```python
from build123d import *

# Parameters (mm, degrees)
BOSS_EXTRUDE1_DEPTH = 10.414
CUT_EXTRUDE1_DEPTH  = 6.08
CUT_EXTRUDE3_DEPTH  = 2.38125
CUT_EXTRUDE2_DEPTH  = 22.784724751


with BuildPart() as part:
    # Sketch1 → Boss-Extrude1 (new body, symmetric)
    with BuildSketch(Plane.XY):
        with BuildLine():
            Line((-1.27, 18.632678954), (-1.27, 14.549677831))
            ThreePointArc((-1.27, 14.549677831), (-10.766948848, 9.86807162), (-14.605, 0))
            Line((-14.605, 0), (-23.054724751, 0))
            Line((-23.054724751, 0), (-23.054724751, 10.414))
            Line((-23.054724751, 10.414), (-16.704724751, 10.414))
            ThreePointArc((-16.704724751, 10.414), (-12.237922792, 15.418575509), (-6.35, 18.632678954))
            Line((-6.35, 18.632678954), (-6.35, 27.522678954))
            Line((-6.35, 27.522678954), (-1.27, 27.522678954))
            Line((-1.27, 27.522678954), (-1.27, 18.632678954))
        make_face()
    boss_extrude1 = extrude(amount=BOSS_EXTRUDE1_DEPTH, both=True)

    # Mirror1: Boss-Extrude1 across plane
    add(boss_extrude1.mirror(Plane(origin=(-23.054724751, 0, 10.414), x_dir=(0, 0, 1), z_dir=(0, 1, 0))))

    # Sketch2 → Cut-Extrude1 (cut, through all)
    with BuildSketch(Plane.ZY.offset(6.35)):
        Polygon((5.207, 25.412545545), (2.872133409, 23.077678954), (5.207, 20.742812362), (7.541866591, 23.077678954), align=None)
        Polygon((-7.541866591, 23.077678954), (-5.207, 20.742812362), (-2.872133409, 23.077678954), (-5.207, 25.412545545), align=None)
    cut_extrude1 = extrude(amount=-CUT_EXTRUDE1_DEPTH, mode=Mode.SUBTRACT)

    # Sketch5 → Cut-Extrude3 (cut)
    with BuildSketch(Plane.ZY.offset(6.35)):
        Polygon((-8.873174209, 23.077678954), (-7.040087105, 19.902678954), (-3.373912895, 19.902678954), (-1.540825791, 23.077678954), (-3.373912895, 26.252678954), (-7.040087105, 26.252678954), align=None)
        Polygon((1.540825791, 23.077678954), (3.373912895, 19.902678954), (7.040087105, 19.902678954), (8.873174209, 23.077678954), (7.040087105, 26.252678954), (3.373912895, 26.252678954), align=None)
    cut_extrude3 = extrude(amount=-CUT_EXTRUDE3_DEPTH, mode=Mode.SUBTRACT)

    # Mirror2: Cut-Extrude1, Cut-Extrude3 across plane
    add(cut_extrude1.mirror(Plane.ZX), mode=Mode.SUBTRACT)
    add(cut_extrude3.mirror(Plane.ZX), mode=Mode.SUBTRACT)

    # Sketch3 → Cut-Extrude2 (cut, through all)
    with BuildSketch(Plane.ZY.offset(23.054724751)):
        Polygon((0, 5.388153673), (-5.388153673, 0), (0, -5.388153673), (5.388153673, 0), align=None)
    extrude(amount=-CUT_EXTRUDE2_DEPTH, mode=Mode.SUBTRACT)


solid = part.part
```
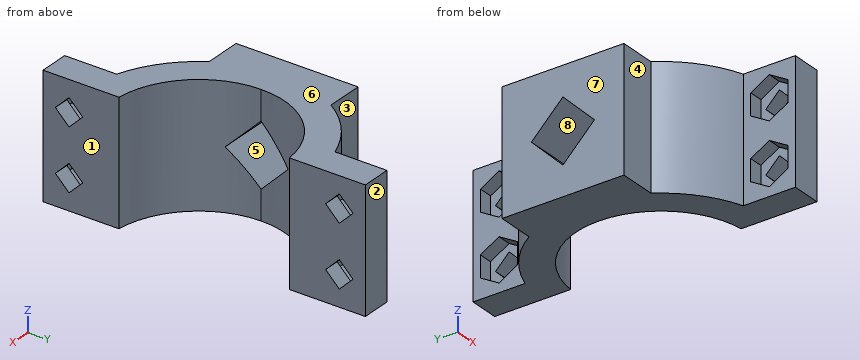
Geometry check sheet. Reference: the model listing, model coordinates, mm. Face numbers are marked on the shaded views. A direction names the side the tool comes from. Coordinates: 2 decimals unless noted, no trailing zeros. Order: outer loops, then holes, each group sorted by start corner. A loop starts at its lowest first (then second) coordinate and runs counter-clockwise, first axis right, second up.
Q1. Tool access check on the marked faces 1, 2, 3, 4 and 5. Record the directions out of +Z, -Z, +X, -X, +Y, -Y that give a thin tool (end or side, any length) a straight path to the whole face; none if there is none.
Reply:
face 1: +Z, -Z, +X, +Y, -Y
face 2: +Z, -Z, +X, -X, +Y
face 3: +Z, -Z, -X, +Y
face 4: +Z, -Z, -X, -Y
face 5: +X, -X
Q2. Sectioned sample at A-A on x = -5. Give the number of separate pieces and of enclosed holes in the cut face, and give its area (3 significant figures).
Reply:
separate pieces: 2
enclosed holes: 4
area: 435 mm2
Q3. Thickness scan on probe 1 along Y at (x, z) = (-2.25, 5.5); probe 2 along Y at (x, z) = (-3.25, -7); probe 3 along Y at (x, z) = (-21.75, -6.5). Record the ranges inside material, lowest first.
Reply:
probe 1: y = -27.52 to -25.12, -21.04 to -14.43, 14.43 to 21.04, 25.12 to 27.52
probe 2: y = -27.52 to -23.62, -22.54 to -14.24, 14.24 to 22.54, 23.62 to 27.52
probe 3: y = -10.41 to 10.41
Q4. Sectioned sample at B-B on y = 3. Record the cut outline in (x, z).
Reply:
outline: (-23.05, -10.41) - (-14.29, -10.41) - (-14.29, -2.39) - (-23.05, -2.39) - close; (-23.05, 2.39) - (-14.29, 2.39) - (-14.29, 10.41) - (-23.05, 10.41) - close
Q5. Draft check along Z on the marked faces 6, 7 and 8. Enter one of: released by +Z, released by -Z, zero draft, split by the parting line, or undercut.
Reply:
face 6: released by +Z
face 7: zero draft
face 8: undercut
Q6. Sectioned sample at D-D on z = -0.75. Record the cut outline in (x, y) (3 decimals), and give its area (3 significant figures).
Reply:
outline: (-23.055, -10.414) - (-16.705, -10.414) arc R19.685 ccw to (-6.35, -18.633) - (-6.35, -27.523) - (-1.27, -27.523) - (-1.27, -14.55) arc R14.605 cw to (-13.849, -4.638) - (-23.055, -4.638) - close; (-23.055, 4.638) - (-13.849, 4.638) arc R14.605 cw to (-1.27, 14.55) - (-1.27, 27.523) - (-6.35, 27.523) - (-6.35, 18.633) arc R19.685 ccw to (-16.705, 10.414) - (-23.055, 10.414) - close
area: 354 mm2
Q7. Sectioned sample at C-C on x = -21.5. Record the cut outline in (y, z), and give its area (3 significant figures).
Reply:
outline: (-10.41, -10.41) - (10.41, -10.41) - (10.41, 10.41) - (-10.41, 10.41) - close; hole (-5.39, 0) - (0, -5.39) - (5.39, 0) - (0, 5.39) - close
area: 376 mm2
Q8. Depth check by flat-ended pin: pin 1 Ø4 at (y, z) = (11, -3) entering from +X; pin 2 Ø5 at (x, z) = (-20, 5) entering from -Y; pin 3 Ø12 at (y, z) = (2, -8) entering from +X. Enter the tip coordinate at first touch or a pass-through.
Reply:
pin 1: stops at x = -6.66
pin 2: stops at y = -10.41
pin 3: stops at x = -12.22
